Could you check a few things on this model? Use its own coordinates, in mm. Face numbers are marked on the shaded views. Round coordinates to 2 decimals unless told otherwise and drop trailing zeros. Write each loop counter-clockwise with the first axis right and the second up, starting at its lowest first coordinate (ties: lowest second). Pieces come first, ordered by that corner, then holes. Notation, with made-up numbers: (31.5, 67.5) - (87.5, 67.5) arc R29 cw to (87.5, 97.5) - close; hole circle Ø8 at (-27, 21). An arc over 180 degrees is marked (long way). Put each result on its own line as item: value.
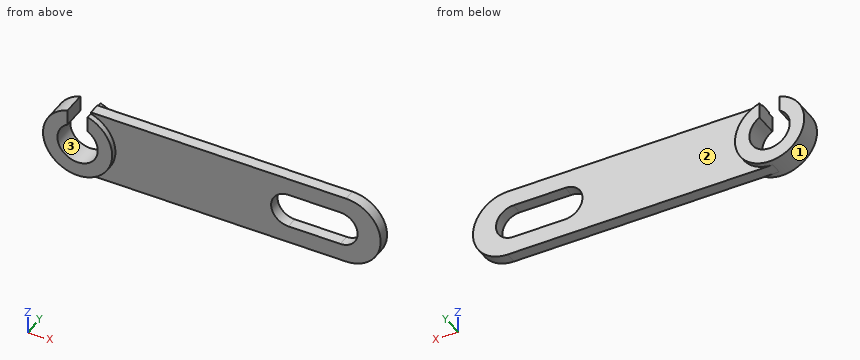
from build123d import *

# Parameters (mm, degrees)
SCHIZZO1_R                    = 1.75
ESTRUSIONE_ESTRUSIONE1_DEPTH  = 0.5
TAGLIO_ESTRUSIONE2_DEPTH      = 15.81553239
TAGLIO_ESTRUSIONE2_DEPTH_BACK = 15.81553239
ESTRUSIONE_ESTRUSIONE2_DEPTH  = 1


with BuildPart() as part:
    # Schizzo1 → Estrusione-Estrusione1 (new, symmetric)
    with BuildSketch(Plane(origin=(0, 0, 0), x_dir=(1, 0, 0), z_dir=(0, 1, 0))):
        with BuildLine():
            Line((-11.5, 3), (11.5, 3))
            ThreePointArc((11.5, 3), (14.5, 0), (11.5, -3))
            Line((11.5, -3), (-11.5, -3))
            ThreePointArc((-11.5, -3), (-14.5, 0), (-11.5, 3))
        make_face()
        with Locations(Location((-11.5, 0, 0), (0, 0, 270))):
            Circle(SCHIZZO1_R, mode=Mode.SUBTRACT)
        with BuildLine():
            Line((11, -1.5), (6.5, -1.5))
            ThreePointArc((6.5, -1.5), (5, 0), (6.5, 1.5))
            Line((6.5, 1.5), (11, 1.5))
            ThreePointArc((11, 1.5), (12.5, 0), (11, -1.5))
        make_face(mode=Mode.SUBTRACT)
    extrude(amount=ESTRUSIONE_ESTRUSIONE1_DEPTH, both=True)

    # Schizzo2 → Taglio-Estrusione2 (cut, two sides: drawn at the far end of the back side and taken through both)
    with BuildSketch(Plane(origin=(0, 0, 0), x_dir=(1, 0, 0), z_dir=(0, 1, 0)).offset(-TAGLIO_ESTRUSIONE2_DEPTH_BACK)):
        with BuildLine():
            Line((-10.625, -1.515544457), (-10.625, -3))
            Line((-10.625, -3), (-11.5, -3))
            ThreePointArc((-11.5, -3), (-11.942334595, -2.967210829), (-12.375, -2.869560071))
            Line((-12.375, -2.869560071), (-12.375, -1.515544457))
            ThreePointArc((-12.375, -1.515544457), (-11.5, -1.75), (-10.625, -1.515544457))
        make_face()
    extrude(amount=TAGLIO_ESTRUSIONE2_DEPTH + TAGLIO_ESTRUSIONE2_DEPTH_BACK, mode=Mode.SUBTRACT)

    # Schizzo4 → Estrusione-Estrusione2 (add, symmetric)
    with BuildSketch(Plane(origin=(0, 0, 0), x_dir=(1, 0, 0), z_dir=(0, 1, 0))):
        with BuildLine():
            Line((-10.625, -2.869560071), (-10.625, -1.515544457))
            ThreePointArc((-10.625, -1.515544457), (-11.5, 1.75), (-12.375, -1.515544457))
            Line((-12.375, -1.515544457), (-12.375, -2.869560071))
            ThreePointArc((-12.375, -2.869560071), (-11.5, 3), (-10.625, -2.869560071))
        make_face()
    extrude(amount=ESTRUSIONE_ESTRUSIONE2_DEPTH, both=True)


solid = part.part
(1) Imagine slicing it at A-A, the plane z = 0. List the corners of the cut face in (x, y) for me.
Values found:
outline: (-14.5, -1) - (-13.25, -1) - (-13.25, 1) - (-14.5, 1) - close; (-9.75, -1) - (-8.5, -1) - (-8.5, -0.5) - (5, -0.5) - (5, 0.5) - (-8.5, 0.5) - (-8.5, 1) - (-9.75, 1) - close; (12.5, -0.5) - (14.5, -0.5) - (14.5, 0.5) - (12.5, 0.5) - close
(2) I'm going to push flat-ended pins straight in: pin 1 (0.7 mm diameter, centred on y = -0.5, z = 2, fed in from +X); pin 2 (3 mm diameter, centred on x = 5.5, z = 0.5, fed in from +Y); pin 3 (1.8 mm diameter, centred on x = 5, z = 0, fed in from -Y); pin 4 (3 mm diameter, centred on x = -11.5, z = 0, fed in from -Y). Where does each tip first touch, or does it pass through?
Values found:
pin 1: stops at x = 14.01
pin 2: stops at y = 0.5
pin 3: stops at y = -0.5
pin 4: passes through
(3) If we mould it in two halves opening along X, with no side actions, what happens to the marked faces 1, 2 and 3? For each: pulls with the +X half, pulls with the -X half, needs draft (parallel to the pull), parting line crosses it, or undercut.
Values found:
face 1: parting line crosses it
face 2: needs draft
face 3: undercut
(4) Imagine slicing it at C-C, the plane y = -0.05. List the corners of the cut face in (x, z) for me (3 decimals).
Values found:
outline: (-12.375, 1.516) - (-12.375, 2.87) arc R3 ccw to (-11.5, -3) - (11.5, -3) arc R3 ccw to (11.5, 3) - (-10.625, 3) - (-10.625, 1.516) arc R1.75 cw (long way) to start; hole (6.5, -1.5) - (11, -1.5) arc R1.5 ccw to (11, 1.5) - (6.5, 1.5) arc R1.5 ccw to start
(5) Imagine slicing it at D-D, the plane z = -1.15. List the corners of the cut face in (x, y) for me, then the cut area to 3 significant figures.
Values found:
outline: (-14.27, -1) - (-12.82, -1) - (-12.82, 1) - (-14.27, 1) - close; (-10.18, -1) - (-8.73, -1) - (-8.73, -0.5) - (5.54, -0.5) - (5.54, 0.5) - (-8.73, 0.5) - (-8.73, 1) - (-10.18, 1) - close; (11.96, -0.5) - (14.27, -0.5) - (14.27, 0.5) - (11.96, 0.5) - close
area: 22.4 mm^2
(6) Please list where these lines run through material, in increasing order: probe 1 along Z at (x, y) = (10.25, -0.25); probe 2 along X at (y, z) = (0.2, 0.7); probe 3 along X at (y, z) = (0.05, 1.25). Write a range as from..to.
Values found:
probe 1: z = -3..-1.5, 1.5..3
probe 2: x = -14.42..-13.1, -9.9..5.17, 12.33..14.42
probe 3: x = -14.23..-12.72, -10.28..5.67, 11.83..14.23
(7) Imagine slicing it at B-B, the plane x = 8.75. List the corners of the cut face in (y, z) for me, then the cut area to 3 significant figures.
Values found:
outline: (-0.5, -3) - (0.5, -3) - (0.5, -1.5) - (-0.5, -1.5) - close; (-0.5, 1.5) - (0.5, 1.5) - (0.5, 3) - (-0.5, 3) - close
area: 3.00 mm^2
